The listing builds one solid part. Answer for the finished solid, in the listing's coordinates (mm). Face numbers are marked on the shaded views. A direction names the side the tool comes from. Round coordinates to 2 decimals unless told otherwise and drop trailing zeros. Write each loop counter-clockwise with the first axis right and the second up, starting at its lowest first coordinate (ties: lowest second). Pieces come first, ordered by that corner, then holes. Notation, with made-up numbers: (42.25, 10) -> (48.25, 10) arc R12 ccw to (48.25, 31) -> close; hole circle Ø4 at (36.5, 68.25). An arc over 180 degrees is marked (long way). Write each question's results on one line, items separated by ' | '. Start each with the question number.
```python
from build123d import *

# Parameters (mm, degrees)
PAD_DEPTH       = 40
POCKET_DEPTH    = 32
POCKET001_DEPTH = 1.5
SKETCH007_R     = 4
SKETCH007_R_2   = 1.95
SKETCH007_R_3   = 2
PAD005_DEPTH    = 6
SKETCH008_W     = 16
SKETCH008_H     = 8
POCKET002_DEPTH = 39
SKETCH013_R     = 1.95
POCKET003_DEPTH = 8
SKETCH018_W     = 39.6
SKETCH018_H     = 12
SKETCH018_H_2   = 9
PAD012_DEPTH    = 17
SKETCH019_W     = 35.9
SKETCH019_H     = 56.1
POCKET006_DEPTH = 11.9
SKETCH023_W     = 79.5
SKETCH023_H     = 6
POCKET007_DEPTH = 0.6


with BuildPart() as part:
    # Sketch → Pad (new body, symmetric)
    with BuildSketch(Plane.XZ):
        Polygon((-49, 17), (-49, -7), (-31, -7), (-31, 0), (49, 0), (49, 17), align=None)
    extrude(amount=PAD_DEPTH, both=True)

    # Sketch001 → Pocket (cut, symmetric)
    with BuildSketch(Plane.XZ):
        Polygon((-32, 1.5), (41, 1.5), (41, 18.5), (-48, 18.5), (-48, -5.5), (-32, -5.5), align=None)
    extrude(amount=POCKET_DEPTH, both=True, mode=Mode.SUBTRACT)

    # Sketch004 → Pocket001 (cut)
    with BuildSketch(Plane.XY):
        with BuildLine():
            ThreePointArc((-3.5, 5), (-8.5, 0), (-3.5, -5))
            Line((-3.5, -5), (21.5, -5))
            ThreePointArc((21.5, -5), (26.5, 0), (21.5, 5))
            Line((21.5, 5), (-3.5, 5))
        make_face()
    extrude(amount=POCKET001_DEPTH, mode=Mode.SUBTRACT)

    # Sketch007 → Pad005 (join)
    with BuildSketch(Plane.XY):
        with Locations((13.1, 14)):
            Circle(SKETCH007_R)
        with Locations((13.1, 14)):
            Circle(SKETCH007_R_2, mode=Mode.SUBTRACT)
        with Locations((35.1, 14)):
            Circle(SKETCH007_R)
        with Locations((35.1, 14)):
            Circle(SKETCH007_R_2, mode=Mode.SUBTRACT)
        with Locations((24.1, -17)):
            Circle(SKETCH007_R_3)
    extrude(amount=PAD005_DEPTH)

    # Sketch008 → Pocket002 (cut, symmetric)
    with BuildSketch(Plane.XZ):
        with Locations((-40, -1.5)):
            Rectangle(SKETCH008_W, SKETCH008_H)
    extrude(amount=POCKET002_DEPTH, both=True, mode=Mode.SUBTRACT)

    # Sketch013 (on DatumPlane) → Pocket003 (cut)
    with BuildSketch(Plane.XY.offset(17)):
        with Locations((-45, 36)):
            Circle(SKETCH013_R)
        with Locations((11, 36)):
            Circle(SKETCH013_R)
        with Locations((45, 36)):
            Circle(SKETCH013_R)
        with Locations((45, -36)):
            Circle(SKETCH013_R)
        with Locations((11, -36)):
            Circle(SKETCH013_R)
        with Locations((-45, -36)):
            Circle(SKETCH013_R)
    extrude(amount=-POCKET003_DEPTH, mode=Mode.SUBTRACT)

    # Sketch018 → Pad012 (join)
    with BuildSketch(Plane.XY):
        with Locations((-12.2, 20.8)):
            Rectangle(SKETCH018_W, SKETCH018_H)
        with Locations((-12.2, -27.5)):
            Rectangle(SKETCH018_W, SKETCH018_H_2)
    extrude(amount=PAD012_DEPTH)

    # Sketch019 (on DatumPlane) → Pocket006 (cut)
    with BuildSketch(Plane.XY.offset(17)):
        with Locations((-12.05, -3.95)):
            Rectangle(SKETCH019_W, SKETCH019_H)
    extrude(amount=-POCKET006_DEPTH, mode=Mode.SUBTRACT)

    # Sketch023 → Pocket007 (cut)
    with BuildSketch(Plane.XY):
        with Locations((8.75, 0)):
            Rectangle(SKETCH023_W, SKETCH023_H)
    extrude(amount=POCKET007_DEPTH, mode=Mode.SUBTRACT)


solid = part.part
```
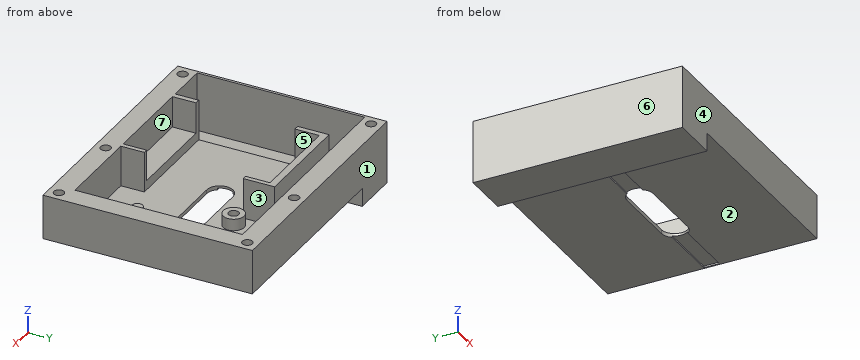
Q1. For the marked faces 1, 2 and 3, determine the directions among +Z, -Z, +X, -X, +Y, -Y from which every point of the face is accessible in a straight line to the end or side of a thin tool.
Q2. The part is cut by section D-D, the plane x = 0. Write down the section's boundary in (y, z).
Q3. Each of these flat-tipped pins is pushed along its axis until it touches: pin 1 (4.5 mm diameter, centred on x = 24.5, y = -16.5, fed in from +Z); pin 2 (4.5 mm diameter, centred on x = 13.1, y = 14, fed in from -Z). Where does it stop, or does it pass through?
Q4. The part is cut by section C-C, the plane y = 36. Write down the section's boundary in (x, z).
Q5. The part is cut by section A-A, the plane z = 7.25. Write down the section's boundary in (x, y).
Q6. Determine the mould class of the marked faces 4, 5, 6 and 7 for opening direction X: pulls with the +X half, pulls with the -X half, needs draft (parallel to the pull), parting line crosses it, or undercut.
Q7. The part is cut by section B-B, the plane y = 0. Write down the section's boundary in (x, z).
Q8. Find the intervals of material crossed by line 1 (X direction, y = 14, z = 3.35); line 2 (X direction, y = 24, z = 2.75); line 3 (Y direction, x = -6, z = 11.25), in increasing order.
Answers follow:
1) face 1: +Z, -Z, +X, -X, +Y | face 2: -Z, +X, +Y, -Y | face 3: +Z
2) outline: (-40, 0) -> (-5, 0) -> (-5, 1.5) -> (-23, 1.5) -> (-23, 5.1) -> (-32, 5.1) -> (-32, 17) -> (-40, 17) -> close; (5, 0) -> (40, 0) -> (40, 17) -> (32, 17) -> (32, 1.5) -> (26.8, 1.5) -> (26.8, 17) -> (24.1, 17) -> (24.1, 5.1) -> (14.8, 5.1) -> (14.8, 1.5) -> (5, 1.5) -> close
3) pin 1: z = 6 | pin 2: z = 0
4) outline: (-49, -7) -> (-31, -7) -> (-31, 0) -> (49, 0) -> (49, 17) -> (46.95, 17) -> (46.95, 9) -> (43.05, 9) -> (43.05, 17) -> (12.95, 17) -> (12.95, 9) -> (9.05, 9) -> (9.05, 17) -> (-43.05, 17) -> (-43.05, 9) -> (-46.95, 9) -> (-46.95, 17) -> (-49, 17) -> close; hole (-48, -5.5) -> (-32, -5.5) -> (-32, 2.5) -> (-48, 2.5) -> close
5) outline: (-49, -40) -> (49, -40) -> (49, 40) -> (-49, 40) -> close; (-32, 14.8) -> (-30, 14.8) -> (-30, 24.1) -> (5.9, 24.1) -> (5.9, 14.8) -> (7.6, 14.8) -> (7.6, 26.8) -> (-32, 26.8) -> close; hole (-48, -32) -> (-32, -32) -> (-32, -23) -> (-30, -23) -> (-30, -32) -> (5.9, -32) -> (5.9, -23) -> (7.6, -23) -> (7.6, -32) -> (41, -32) -> (41, 32) -> (-48, 32) -> close
6) face 4: needs draft | face 5: undercut | face 6: pulls with the -X half | face 7: undercut
7) outline: (-49, -7) -> (-31, -7) -> (-31, 0.6) -> (-8.5, 0.6) -> (-8.5, 1.5) -> (-32, 1.5) -> (-32, -5.5) -> (-48, -5.5) -> (-48, 17) -> (-49, 17) -> close; (26.5, 0.6) -> (48.5, 0.6) -> (48.5, 0) -> (49, 0) -> (49, 17) -> (41, 17) -> (41, 1.5) -> (26.5, 1.5) -> close
8) line 1: -49 to -48, 9.1 to 11.15, 15.05 to 17.1, 31.1 to 33.15, 37.05 to 39.1, 41 to 49 | line 2: -49 to -48, -32 to 7.6, 41 to 49 | line 3: -40 to -32, 24.1 to 26.8, 32 to 40
